The listing builds one solid part. Answer for the finished solid, in the listing's coordinates (mm). Coordinates: 2 decimals unless noted, no trailing zeros. Order: outer loops, then holes, each group sorted by start corner. A loop starts at its lowest first (then second) coordinate and runs counter-clockwise, first axis right, second up. Notation, with made-up numbers: (-0.5, -8.75) - (29.5, -8.75) arc R22 cw to (29.5, 1.25) - close; hole circle Ø9 at (-31, 54). An arc over 180 degrees is marked (long way). Use one line per item in the form item = value. Start each with the question number.
Item 1: Section B-B, the plane y = 2.5 is taken. Write down the section's boundary in (x, z).
Item 2: This flat-tipped pin is pushed along its axis until it touches: pin 1 Ø3 at (y, z) = (2.5, 2) entering from -X. Where does it stop, or does it pass through?
Item 3: The mould has two halves that part along X. Classify faces 1 (the cylindrical face through (-1.76, -2.99, 2.46)), 2 (the cylindrical face through (-1.719, 3.037, 2.465)), 3 (the flat face through (0, 0, 5)): released by +X, released by -X, zero draft, split by the parting line, or undercut.
Item 4: Section A-A, the plane x = 2.25 is taken. Write down the section's boundary in (y, z).
Item 5: Section D-D, the plane x = -1.75 is taken. Write down the section's boundary in (y, z), and give its area (3 significant figures).
Item 6: Consider line 1 along X through (y, z) = (3, 1.4); line 2 along X through (y, z) = (-2.25, 0.9); line 3 along Y through (x, z) = (3.25, 2.35). Determine where each line is inside the solid, lowest interval first. Write a range as [from, to].
from build123d import *

# Parameters (mm, degrees)
F1_DEPTH = 5


with BuildPart() as f1:
    # F0 (on Top) → F1 (new body)
    with BuildSketch(Plane.XY):
        with BuildLine():
            ThreePointArc((-0.0032454835, 2.4100617583), (-1.7444594295, 3.0227098771), (-2.115982294, 1.2146350766))
            ThreePointArc((-2.115982294, 1.2146350766), (-1.660800532, 1.0598981147), (-1.3002209241, 0.7419102056))
            ThreePointArc((-1.3002209241, 0.7419102056), (-0.5166175034, 0.9027342531), (0.0006491683, 1.5129259324))
            ThreePointArc((0.0006491683, 1.5129259324), (-0.0863815539, 1.9611244808), (-0.0032454835, 2.4100617583))
        make_face()
        with BuildLine():
            ThreePointArc((-2.115982294, 1.2146350766), (-3.083031036, 0.9207121401), (-3.5, 0))
            ThreePointArc((-3.5, 0), (-3.0790448546, -0.9241952563), (-2.1054908215, -1.213215413))
            ThreePointArc((-2.1054908215, -1.213215413), (-1.7471466082, -0.8904039187), (-1.2919668901, -0.7309383728))
            ThreePointArc((-1.2919668901, -0.7309383728), (-1.1120639399, -0.3849736616), (-1.05, 0))
            ThreePointArc((-1.05, 0), (-1.1142396096, 0.3914847583), (-1.3002209241, 0.7419102056))
            ThreePointArc((-1.3002209241, 0.7419102056), (-1.7554026862, 0.8966471675), (-2.115982294, 1.2146350766))
        make_face()
        with BuildLine():
            ThreePointArc((-1.3002209241, 0.7419102056), (-1.660800532, 1.0598981147), (-2.115982294, 1.2146350766))
            ThreePointArc((-2.115982294, 1.2146350766), (-1.7554026862, 0.8966471675), (-1.3002209241, 0.7419102056))
        make_face()
        with BuildLine():
            ThreePointArc((-1.2919668901, -0.7309383728), (-1.7471466082, -0.8904039187), (-2.1054908215, -1.213215413))
            ThreePointArc((-2.1054908215, -1.213215413), (-1.6503111034, -1.0537498671), (-1.2919668901, -0.7309383728))
        make_face()
        with BuildLine():
            ThreePointArc((-1.2919668901, -0.7309383728), (-1.6503111034, -1.0537498671), (-2.1054908215, -1.213215413))
            ThreePointArc((-2.1054908215, -1.213215413), (-1.7359979287, -3.0044336554), (0.0011148123, -2.4322211823))
            ThreePointArc((0.0011148123, -2.4322211823), (-0.0939762845, -1.9509044509), (0.0074248045, -1.4708774395))
            ThreePointArc((0.0074248045, -1.4708774395), (-0.5162756494, -0.8796500011), (-1.2919668901, -0.7309383728))
        make_face()
        with BuildLine():
            ThreePointArc((2.3559973284, -1.958944836), (2.2909030568, -1.5649350629), (2.1025382242, -1.212799215))
            ThreePointArc((2.1025382242, -1.212799215), (1.6572404008, -1.0578270547), (1.3034591042, -0.746145621))
            ThreePointArc((1.3034591042, -0.746145621), (0.5331160977, -0.8897568104), (0.0074248045, -1.4708774395))
            ThreePointArc((0.0074248045, -1.4708774395), (0.0785275261, -1.702783823), (0.1025422884, -1.9441537858))
            ThreePointArc((0.1025422884, -1.9441537858), (0.0769174053, -2.1934013116), (0.0011148123, -2.4322211823))
            ThreePointArc((0.0011148123, -2.4322211823), (1.3723672911, -3.1599300737), (2.3559973284, -1.958944836))
        make_face()
        with BuildLine():
            ThreePointArc((2.1025382242, -1.212799215), (3.0779194619, -0.9251731393), (3.5, 0))
            ThreePointArc((3.5, 0), (3.0786929463, 0.9245012969), (2.1045671053, 1.2130859938))
            ThreePointArc((2.1045671053, 1.2130859938), (1.7515384972, 0.905810587), (1.3090397977, 0.7533564147))
            ThreePointArc((1.3090397977, 0.7533564147), (1.0500084837, 0.0045590483), (1.3034591042, -0.746145621))
            ThreePointArc((1.3034591042, -0.746145621), (1.7487569276, -0.9011177813), (2.1025382242, -1.212799215))
        make_face()
        with BuildLine():
            ThreePointArc((1.3090397977, 0.7533564147), (1.6620684058, 1.0606318215), (2.1045671053, 1.2130859938))
            ThreePointArc((2.1045671053, 1.2130859938), (2.2970382233, 1.5681185753), (2.363606903, 1.9664424086))
            ThreePointArc((2.363606903, 1.9664424086), (1.3642790397, 3.170476082), (-0.0032454835, 2.4100617583))
            ThreePointArc((-0.0032454835, 2.4100617583), (0.0618394297, 2.1874422019), (0.0837967819, 1.9565452822))
            ThreePointArc((0.0837967819, 1.9565452822), (0.0628304553, 1.7308731455), (0.0006491683, 1.5129259324))
            ThreePointArc((0.0006491683, 1.5129259324), (0.5235763818, 0.9070263156), (1.3090397977, 0.7533564147))
        make_face()
        with BuildLine():
            ThreePointArc((0.0837967819, 1.9565452822), (0.0618394297, 2.1874422019), (-0.0032454835, 2.4100617583))
            ThreePointArc((-0.0032454835, 2.4100617583), (-0.0863815539, 1.9611244808), (0.0006491683, 1.5129259324))
            ThreePointArc((0.0006491683, 1.5129259324), (0.0628304553, 1.7308731455), (0.0837967819, 1.9565452822))
        make_face()
        with BuildLine():
            ThreePointArc((1.3090397977, 0.7533564147), (1.7515384972, 0.905810587), (2.1045671053, 1.2130859938))
            ThreePointArc((2.1045671053, 1.2130859938), (1.6620684058, 1.0606318215), (1.3090397977, 0.7533564147))
        make_face()
        with BuildLine():
            ThreePointArc((1.3034591042, -0.746145621), (1.6572404008, -1.0578270547), (2.1025382242, -1.212799215))
            ThreePointArc((2.1025382242, -1.212799215), (1.7487569276, -0.9011177813), (1.3034591042, -0.746145621))
        make_face()
        with BuildLine():
            ThreePointArc((0.0074248045, -1.4708774395), (-0.0939762845, -1.9509044509), (0.0011148123, -2.4322211823))
            ThreePointArc((0.0011148123, -2.4322211823), (0.0769174053, -2.1934013116), (0.1025422884, -1.9441537858))
            ThreePointArc((0.1025422884, -1.9441537858), (0.0785275261, -1.702783823), (0.0074248045, -1.4708774395))
        make_face()
        with BuildLine():
            ThreePointArc((1.3034591042, -0.746145621), (1.0500084837, 0.0045590483), (1.3090397977, 0.7533564147))
            ThreePointArc((1.3090397977, 0.7533564147), (0.5235763818, 0.9070263156), (0.0006491683, 1.5129259324))
            ThreePointArc((0.0006491683, 1.5129259324), (-0.5166175034, 0.9027342531), (-1.3002209241, 0.7419102056))
            ThreePointArc((-1.3002209241, 0.7419102056), (-1.1142396096, 0.3914847583), (-1.05, 0))
            ThreePointArc((-1.05, 0), (-1.1120639399, -0.3849736616), (-1.2919668901, -0.7309383728))
            ThreePointArc((-1.2919668901, -0.7309383728), (-0.5162756494, -0.8796500011), (0.0074248045, -1.4708774395))
            ThreePointArc((0.0074248045, -1.4708774395), (0.5331160977, -0.8897568104), (1.3034591042, -0.746145621))
        make_face()
    extrude(amount=F1_DEPTH)


solid = f1.part
Response:
q1.outline = (-2.24, 0) - (-0.04, 0) - (-0.04, 5) - (-2.24, 5) - close; (0.04, 0) - (2.24, 0) - (2.24, 5) - (0.04, 5) - close
q2.pin_1 = -2.98
q3.face_1 = undercut
q3.face_2 = undercut
q3.face_3 = zero draft
q4.outline = (-2.46, 0) - (-1.46, 0) - (-1.46, 5) - (-2.46, 5) - close; (-1.22, 0) - (1.22, 0) - (1.22, 5) - (-1.22, 5) - close; (1.45, 0) - (2.48, 0) - (2.48, 5) - (1.45, 5) - close
q5.outline = (-3, 0) - (3.02, 0) - (3.02, 5) - (-3, 5) - close
q5.area = 30.1 mm2
q6.line_1 = [-1.78, -0.5], [0.48, 1.8]
q6.line_2 = [-2.31, 2.32]
q6.line_3 = [-0.74, 0.74]
